Can you work these out from the drawing? Everything is in mm from the part's minimum corner. A direction names the side the tool comes from. Give positions to 0.01 mm unless a question says otherwise; leave off trailing zeros. Order: outer loops, then holes, each group sorted by start corner. A loop starts at its lowest first (then second) coordinate and runs counter-clockwise, first axis right, second up. Notation, with made-up numbers: (-1, 87.5) - (55, 87.5) arc R23 ccw to (55, 110.5) - close; hole circle Ø11 at (68, 57). An arc over 180 degrees is marked (long way). One line per question, with ' | ' between items.
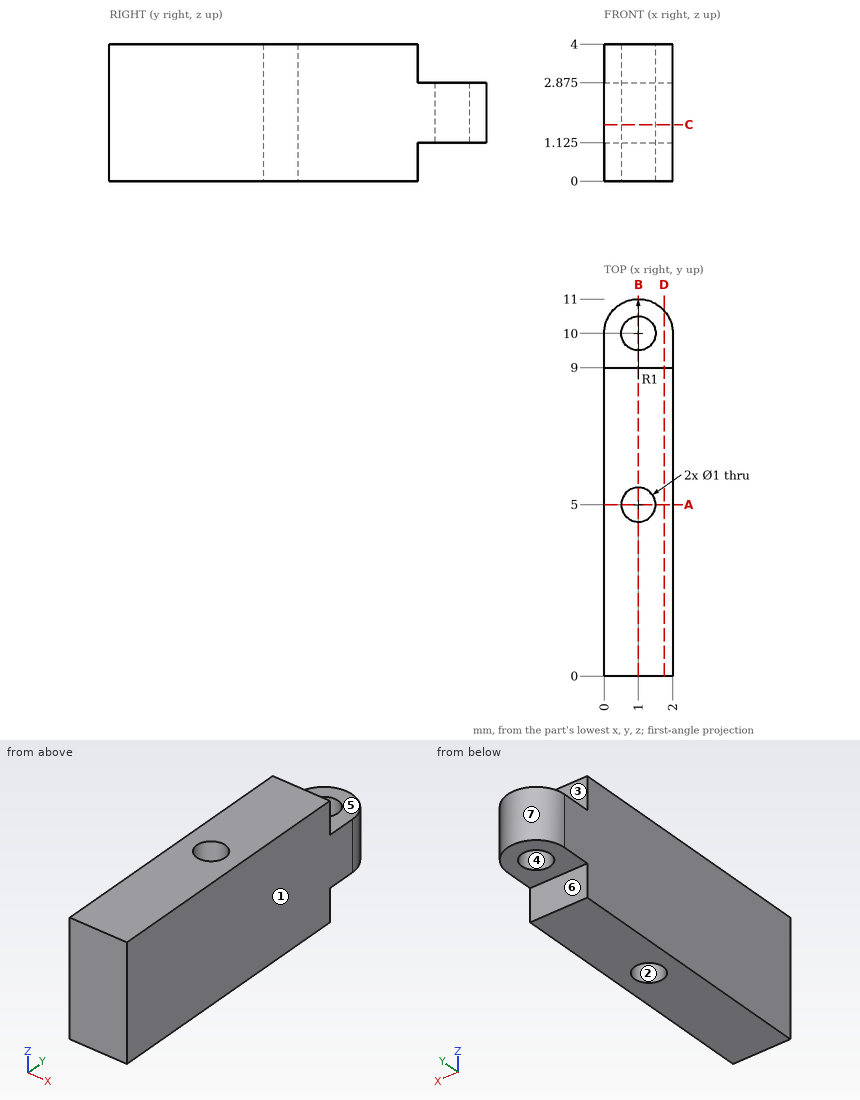
1) Please list where these lines run through material, in increasing order: L1, parallel to Y at x = 1, z = 1.5; L2, parallel to X at y = 10, z = 1.5; L3, parallel to Y at x = 0.75, z = 2.4.
Model answer:
L1: y = 0 to 4.5, 5.5 to 9.5, 10.5 to 11 | L2: x = 0 to 0.5, 1.5 to 2 | L3: y = 0 to 4.57, 5.43 to 9.57, 10.43 to 10.97
2) Thinking about a two-plate mould opening in X: for the marked faces 1, 2, 3 and 4, which applies, +X half, -X half, draft (parallel to the pull), parting line (faces both ways), or undercut?
Model answer:
face 1: +X half | face 2: undercut | face 3: draft | face 4: undercut
3) I want a section at D-D (x = 1.75). List the corners of the cut face in (y, z) for me (3 decimals), plus the area to 3 significant figures.
Model answer:
outline: (0, 0) - (9, 0) - (9, 1.125) - (10.661, 1.125) - (10.661, 2.875) - (9, 2.875) - (9, 4) - (0, 4) - close | area: 38.9 mm2
4) I'm going to push flat-ended pins straight in: P1, Ø0.6, axis at x = 0.5, y = 10, coming from the +Z side (3 decimals); P2, Ø0.6, axis at x = 1.5, y = 10, coming from the -Z side (3 decimals). Where does each tip first touch, or does it pass through?
Model answer:
P1: stops at z = 2.875 | P2: stops at z = 1.125
5) I want a section at C-C (z = 1.65). List the corners of the cut face in (x, y) for me, plus the area to 3 significant figures.
Model answer:
outline: (0, 0) - (2, 0) - (2, 10) arc R1 ccw to (0, 10) - close; hole circle Ø1 at (1, 5); hole circle Ø1 at (1, 10) | area: 20.0 mm2
6) On a 3-axis mill with a long thin cutter (end or side, diameter ignored), from which of +Z, -Z, +X, -X, +Y, -Y can I reach the whole of each face in a straight line? I mean the marked faces 5, 6 and 7. Say none if no direction works.
Model answer:
face 5: +Z, +X, -X, +Y | face 6: -Z, +X, -X, +Y | face 7: +Z, -Z, +Y
7) I want a section at B-B (x = 1). List the corners of the cut face in (y, z) for me (3 decimals).
Model answer:
outline: (0, 0) - (4.5, 0) - (4.5, 4) - (0, 4) - close; (5.5, 0) - (9, 0) - (9, 1.125) - (9.5, 1.125) - (9.5, 2.875) - (9, 2.875) - (9, 4) - (5.5, 4) - close; (10.5, 1.125) - (11, 1.125) - (11, 2.875) - (10.5, 2.875) - close
8) I want a section at A-A (y = 5). List the corners of the cut face in (x, z) for me.
Model answer:
outline: (0, 0) - (0.5, 0) - (0.5, 4) - (0, 4) - close; (1.5, 0) - (2, 0) - (2, 4) - (1.5, 4) - close
